The listing builds one solid part. Answer for the finished solid, in the listing's coordinates (mm). A direction names the side the tool comes from. Give positions to 0.01 mm unless a question says otherwise; leave off trailing zeros. Write each loop counter-clockwise with the first axis right and the second up, starting at its lowest first coordinate (ties: lowest second). Pieces come first, ordered by that corner, then holes. Notation, with made-up numbers: (50, -8) - (74, -8) arc R21 cw to (74, 0) - close; hole circle Ø4 at (20, -24.5). An arc over 180 degrees is marked (long way). One line per question, with ' | ' between items. Start each with the question number.
1. A cutting plane is placed at B-B (y = -7). Determine the outline of the cut face in (x, z).
2. Find the intervals of material crossed by L1, parallel to Y at x = 0, z = 0.3; L2, parallel to Y at x = 0, z = 1.25; L3, parallel to Z at x = -0.5, y = 2.5, in increasing order. Write a range as from..to.
3. Given P1, Ø1.8, axis at x = 0, y = 0, coming from the +Z side; P2, Ø5, axis at x = 0, y = 0, coming from the +Z side; P3, Ø1.5, axis at y = -2.5, z = 0.5, coming from the -X side; P4, Ø1, axis at x = 5, z = 1.5, coming from the +Y side, each flat-ended and moving along its own axis, determine where each tip first touches the part or whether it passes through.
4. A cutting plane is placed at A-A (x = 8). Determine the outline of the cut face in (y, z).
5. The mould has two halves that part along Y. Classify faces 3 (the face through (-0.325, -8.464, 0.887)), 4 (the face through (-0.943, -4.247, 3.18)), 5 (the face through (-3, 0, 4.6)): +Y half, -Y half, draft (parallel to the pull), parting line (faces both ways), or undercut.
6. For faces 1 (the face through (1.3, 1.4, 1.1)), 2 (the face through (0, -2, 0)), determine the directions among +Z, -Z, +X, -X, +Y, -Y from which every point of the face is accessible in a straight line to the end or side of a thin tool.
```python
from build123d import *

# Parameters (mm, degrees)
SKETCH1_R           = 10
SKETCH1_R_2         = 1.5
SKETCH1_R_3         = 4.35
BOSS_EXTRUDE1_DEPTH = 1.8
SKETCH1_2_R         = 4.35
BOSS_EXTRUDE2_DEPTH = 4.6
SKETCH2_R           = 1.5
CUT_EXTRUDE1_DEPTH  = 4.5
SKETCH3_R           = 2.75
CUT_EXTRUDE2_DEPTH  = 3.5
CUT_EXTRUDE3_DEPTH  = 3.5
CIRPATTERN1_COUNT   = 25


with BuildPart() as part:
    # Sketch1 → Boss-Extrude1 (new body)
    with BuildSketch(Plane.XY):
        Circle(SKETCH1_R)
        with Locations((0, 7)):
            Circle(SKETCH1_R_2, mode=Mode.SUBTRACT)
        with Locations((7, 0)):
            Circle(SKETCH1_R_2, mode=Mode.SUBTRACT)
        with Locations((0, -7)):
            Circle(SKETCH1_R_2, mode=Mode.SUBTRACT)
        with Locations((-7, 0)):
            Circle(SKETCH1_R_2, mode=Mode.SUBTRACT)
        Circle(SKETCH1_R_3, mode=Mode.SUBTRACT)
    extrude(amount=BOSS_EXTRUDE1_DEPTH)

    # Sketch1_2 → Boss-Extrude2 (add)
    with BuildSketch(Plane.XY):
        Circle(SKETCH1_2_R)
    extrude(amount=BOSS_EXTRUDE2_DEPTH)

    # Sketch2 → Cut-Extrude1 (cut)
    with BuildSketch(Plane(origin=(0, 0, 0), x_dir=(-1, 0, 0), z_dir=(0, 0, -1))):
        Circle(SKETCH2_R)
    extrude(amount=-CUT_EXTRUDE1_DEPTH, mode=Mode.SUBTRACT)

    # Sketch3 → Cut-Extrude2 (cut)
    with BuildSketch(Plane.XY.offset(4.6)):
        Circle(SKETCH3_R)
    extrude(amount=-CUT_EXTRUDE2_DEPTH, mode=Mode.SUBTRACT)

    # Sketch4 → Cut-Extrude3 (cut)
    with BuildSketch(Plane.XY.offset(4.6)):
        with BuildLine():
            Line((-2.976344104, 0.375999701), (-2.728315429, 0.344666392))
            ThreePointArc((-2.728315429, 0.344666392), (-2.70218519, 0.510583192), (-2.665974712, 0.674595311))
            Line((-2.665974712, 0.674595311), (-2.976344104, 0.375999701))
        make_face()
        with BuildLine():
            Line((-2.976344104, 0.375999701), (-2.75, 0))
            ThreePointArc((-2.75, 0), (-2.744573503, 0.172673929), (-2.728315429, 0.344666392))
            Line((-2.728315429, 0.344666392), (-2.976344104, 0.375999701))
        make_face()
    cut_extrude3 = extrude(amount=-CUT_EXTRUDE3_DEPTH, mode=Mode.SUBTRACT)

    # CirPattern1: Cut-Extrude3 ×25 about axis
    cirpattern1_axis = Axis((0, 0, 0), (0, 0, 1))
    for i in range(1, CIRPATTERN1_COUNT):
        add(cut_extrude3.rotate(cirpattern1_axis, i * 360 / CIRPATTERN1_COUNT), mode=Mode.SUBTRACT)


solid = part.part
```
Determined:
1) outline: (-7.14, 0) - (-1.5, 0) - (-1.5, 1.8) - (-7.14, 1.8) - close; (1.5, 0) - (7.14, 0) - (7.14, 1.8) - (1.5, 1.8) - close
2) L1: -10..-8.5, -5.5..-1.5, 1.5..5.5, 8.5..10 | L2: -10..-8.5, -5.5..-2.86, 2.86..5.5, 8.5..10 | L3: 0..1.1
3) P1: through | P2: z = 1.1 | P3: x = -9.85 | P4: y = 8.93
4) outline: (-6, 0) - (-1.12, 0) - (-1.12, 1.8) - (-6, 1.8) - close; (1.12, 0) - (6, 0) - (6, 1.8) - (1.12, 1.8) - close
5) face 3: undercut | face 4: parting line | face 5: draft
6) face 1: +Z | face 2: -Z, +X, -X, +Y, -Y
